Source: CAD feature listing. Evaluate the final solid. Frame: model axes, mm. Give positions to 0.01 mm unless a question says otherwise; leave off trailing zeros. Order: outer loops, then holes, each group sorted by start corner. A loop starts at its lowest first (then second) coordinate and runs counter-clockwise, first axis right, second up.
```python
from build123d import *

# Parameters (mm, degrees)
F0_R     = 25
F1_DEPTH = 25


with BuildPart() as f1:
    # F0 (on Front) → F1 (new body)
    with BuildSketch(Plane.XZ):
        with BuildLine():
            ThreePointArc((47.017566, 17.010247), (49.248748, 8.634863), (50, 0))
            ThreePointArc((50, 0), (-8.634862, -49.248748), (-47.017566, 17.010246))
            Line((-47.017566, 17.010246), (-140, -240))
            Line((-140, -240), (0, -240))
            Line((0, -240), (140, -240))
            Line((140, -240), (47.017566, 17.010247))
        make_face()
        with BuildLine():
            ThreePointArc((-47.017566, 17.010246), (-8.634862, -49.248748), (50, 0))
            ThreePointArc((50, 0), (49.248748, 8.634863), (47.017566, 17.010247))
            ThreePointArc((47.017566, 17.010247), (-1e-06, 50), (-47.017566, 17.010246))
        make_face()
        Circle(F0_R, mode=Mode.SUBTRACT)
    extrude(amount=F1_DEPTH)


solid = f1.part
```
1) Draft query along Z for faces 1 (the flat face through (-2, -12, -240)), 2 (the cylindrical face through (23.846, -12.325, 7.509)), 3 (the flat face through (-2, -25, -125)), 4 (the flat face through (-92.86, -12.32, -109.7)). Return one class per face: +Z half, -Z half, draft (parallel to the pull), parting line (faces both ways), or undercut.
Report:
face 1: -Z half
face 2: undercut
face 3: draft
face 4: +Z half
2) Pin query (flat end, axial travel): pin 1 (5 mm diameter, centred on y = -7, z = -41, fed in from -X); pin 2 (12 mm diameter, centred on x = 20, y = -5.5, fed in from +Z); pin 3 (12 mm diameter, centred on y = -11, z = -67.5, fed in from +X). Return the tip coordinate at first contact, or that it passes through.
Report:
pin 1: stops at x = -68.91
pin 2: stops at z = 48
pin 3: stops at x = 79.76
3) Section query D-D, the plane z = -219.5. Return the cut outline in (x, y).
Report:
outline: (-132.58, -25) - (132.58, -25) - (132.58, 0) - (-132.58, 0) - close
4) Section query A-A, the plane x = 0. Return the cut outline in (y, z), and give its area (3 significant figures).
Report:
outline: (-25, -240) - (0, -240) - (0, -25) - (-25, -25) - close; (-25, 25) - (0, 25) - (0, 50) - (-25, 50) - close
area: 6,000 mm2
5) Section query C-C, the plane y = -11.25. Return the cut outline in (x, z).
Report:
outline: (-140, -240) - (140, -240) - (47.02, 17.01) arc R50 ccw to (-47.02, 17.01) - close; hole circle Ø50 at (0, 0)
6) Material intervals for L1, parallel to Z at x = 0, y = -16; L2, parallel to X at y = -18, z = 20.5; L3, parallel to X at y = -9, z = 2.5, sorted ascending.
Report:
L1: z = -240 to -25, 25 to 50
L2: x = -45.6 to -14.31, 14.31 to 45.6
L3: x = -52.27 to -24.87, 24.87 to 52.27
7) Section query B-B, the plane z = 0. Return the cut outline in (x, y), and give its area (3 significant figures).
Report:
outline: (-53.17, -25) - (-25, -25) - (-25, 0) - (-53.17, 0) - close; (25, -25) - (53.17, -25) - (53.17, 0) - (25, 0) - close
area: 1,410 mm2
